For this review, take the finished solid that the model builds, in its own axes (mm). Face numbers are marked on the shaded views. A direction names the side the tool comes from. Coordinates: 2 decimals unless noted, no trailing zeros. Order: outer loops, then holes, each group sorted by start corner. A loop starts at its lowest first (then second) coordinate and runs counter-clockwise, first axis right, second up. Notation, with made-up numbers: (45, -18) -> (53, -18) arc R16 ccw to (53, -3) -> close; hole circle Ø10 at (-24, 32.25). An arc over 180 degrees is marked (long way). Write item = value, one per line. Start each with the question number.
1) Wall thickness on probe 1 along X at (y, z) = (-66, -23.48); probe 2 along Y at (x, z) = (-6, -32); probe 3 along Y at (x, z) = (23, 32): over which ranges is each line inside the solid? List them lowest first. Write a range as [from, to].
2) Consider section B-B on z = -23.48. Give the boundary of the cut face in (x, y).
3) Consider section A-A on x = 25. Give the boundary of the cut face in (y, z).
4) Draft analysis for pull direction Y (two halves, no side actions). For the marked faces 1, 2, 3 and 4, state which applies: +Y half, -Y half, draft (parallel to the pull), parting line (faces both ways), or undercut.
5) Consider section D-D on z = -38.5. Give the boundary of the cut face in (x, y).
6) Machinability: for the marked faces 5, 6 and 7, which of the approach directions +Z, -Z, +X, -X, +Y, -Y give a long, thin tool a straight path to every point of the face, cutting with its end or side? Answer none if there is none.
7) Insertion check: pin 1 Ø3 at (x, z) = (7.5, 7.5) entering from -Y; pin 2 Ø1.6 at (y, z) = (-21, -52.5) entering from +X; pin 3 Ø5.5 at (x, y) = (0, -77) entering from -Z. Each pin has a flat end and moves straight along its axis. Give the tip position at first contact, or say it passes through.
8) Consider section C-C on y = -77. Give the boundary of the cut face in (x, z).
from build123d import *

# Parameters (mm, degrees)
SKETCH1_W           = 68
SKETCH1_H           = 107
BOSS_EXTRUDE1_DEPTH = 2
SKETCH2_W           = 68
SKETCH2_H           = 2
BOSS_EXTRUDE2_DEPTH = 67
CUT_EXTRUDE2_REACH  = 132.744
SKETCH4_W           = 11.5
SKETCH4_H           = 15
SKETCH4_W_2         = 38
SKETCH4_H_2         = 21
SKETCH5_W           = 68
SKETCH5_H           = 2
BOSS_EXTRUDE3_DEPTH = 51
SKETCH6_W           = 68
SKETCH6_H           = 2
BOSS_EXTRUDE4_DEPTH = 15
BOSS_EXTRUDE5_DEPTH = 1.5
CUT_EXTRUDE4_REACH  = 96.449
SKETCH9_R           = 1.75
FILLET1_R           = 1.5
FILLET2_R           = 3
FILLET3_R           = 1.5
FILLET4_R           = 3
FILLET5_R           = 1.5
FILLET6_R           = 3
CUT_EXTRUDE5_REACH  = 106.585
SKETCH10_R          = 1.75
CHAMFER1_SIZE       = 2


with BuildPart() as part:
    # Sketch1 → Boss-Extrude1 (new body)
    with BuildSketch(Plane(origin=(0, 0, 0), x_dir=(1, 0, 0), z_dir=(0, 1, 0))):
        Rectangle(SKETCH1_W, SKETCH1_H)
    extrude(amount=BOSS_EXTRUDE1_DEPTH)

    # Sketch2 → Boss-Extrude2 (add)
    with BuildSketch(Plane.XZ):
        with Locations((0, -52.5)):
            Rectangle(SKETCH2_W, SKETCH2_H)
    extrude(amount=BOSS_EXTRUDE2_DEPTH)

    # Sketch4 → Cut-Extrude2 (cut, up to next)
    with BuildSketch(Plane(origin=(0, 0, -53.5), x_dir=(-1, 0, 0), z_dir=(0, 0, -1)), mode=Mode.PRIVATE) as cut_extrude2_sk1:
        with Locations((-25.25, -28)):
            Rectangle(SKETCH4_W, SKETCH4_H)
    cut_extrude2_tool1 = extrude(cut_extrude2_sk1.sketch, amount=-CUT_EXTRUDE2_REACH, mode=Mode.PRIVATE) & part.part
    # Sketch4 → Cut-Extrude2 (cut, up to next)
    with BuildSketch(Plane(origin=(0, 0, -53.5), x_dir=(-1, 0, 0), z_dir=(0, 0, -1)), mode=Mode.PRIVATE) as cut_extrude2_sk2:
        with Locations((9.546940835, -25.7)):
            Rectangle(SKETCH4_W_2, SKETCH4_H_2)
    cut_extrude2_tool2 = extrude(cut_extrude2_sk2.sketch, amount=-CUT_EXTRUDE2_REACH, mode=Mode.PRIVATE) & part.part
    add(cut_extrude2_tool1.solids().sort_by_distance((25.25, -28, -53.5))[0], mode=Mode.SUBTRACT)
    add(cut_extrude2_tool2.solids().sort_by_distance((-9.546941, -25.7, -53.5))[0], mode=Mode.SUBTRACT)

    # Sketch5 → Boss-Extrude3 (add)
    with BuildSketch(Plane.XY.offset(-51.5)):
        with Locations((0, -66)):
            Rectangle(SKETCH5_W, SKETCH5_H)
    extrude(amount=BOSS_EXTRUDE3_DEPTH)

    # Sketch6 → Boss-Extrude4 (add)
    with BuildSketch(Plane.XZ.offset(67)):
        with Locations((0, -1.5)):
            Rectangle(SKETCH6_W, SKETCH6_H)
    extrude(amount=BOSS_EXTRUDE4_DEPTH)

    # Sketch8 → Boss-Extrude5 (add)
    with BuildSketch(Plane(origin=(0, 2, 0), x_dir=(1, 0, 0), z_dir=(0, 1, 0))):
        Polygon((-34.8, 50.5), (-34, 50.5), (-34, -53.5), (34, -53.5), (34, 50.5), (34.8, 50.5), (34.8, -54.3), (-34.8, -54.3), align=None)
    extrude(amount=-BOSS_EXTRUDE5_DEPTH)

    # Sketch9 → Cut-Extrude4 (cut, up to next)
    with BuildSketch(Plane.XZ.offset(67), mode=Mode.PRIVATE) as cut_extrude4_sk1:
        with Locations(Location((-25, -23.48, 0), (0, 0, 270))):
            Circle(SKETCH9_R)
    cut_extrude4_tool1 = extrude(cut_extrude4_sk1.sketch, amount=-CUT_EXTRUDE4_REACH, mode=Mode.PRIVATE) & part.part
    # Sketch9 → Cut-Extrude4 (cut, up to next)
    with BuildSketch(Plane.XZ.offset(67), mode=Mode.PRIVATE) as cut_extrude4_sk2:
        with Locations(Location((25, -23.48, 0), (0, 0, 270))):
            Circle(SKETCH9_R)
    cut_extrude4_tool2 = extrude(cut_extrude4_sk2.sketch, amount=-CUT_EXTRUDE4_REACH, mode=Mode.PRIVATE) & part.part
    add(cut_extrude4_tool1.solids().sort_by_distance((-25, -67, -23.48))[0], mode=Mode.SUBTRACT)
    add(cut_extrude4_tool2.solids().sort_by_distance((25, -67, -23.48))[0], mode=Mode.SUBTRACT)

    # Fillet1
    fillet1_edges = [part.edges().sort_by_distance(p)[0] for p in [
        (0, -67, -2.5),
    ]]
    fillet(fillet1_edges, radius=FILLET1_R)

    # Fillet2
    fillet2_edges = [part.edges().sort_by_distance(p)[0] for p in [
        (0, -65, -0.5),
    ]]
    fillet(fillet2_edges, radius=FILLET2_R)

    # Fillet3
    fillet3_edges = [part.edges().sort_by_distance(p)[0] for p in [
        (0, -65, -51.5),
    ]]
    fillet(fillet3_edges, radius=FILLET3_R)

    # Fillet4
    fillet4_edges = [part.edges().sort_by_distance(p)[0] for p in [
        (0, -67, -53.5),
    ]]
    fillet(fillet4_edges, radius=FILLET4_R)

    # Fillet5
    fillet5_edges = [part.edges().sort_by_distance(p)[0] for p in [
        (0, 0, -51.5),
    ]]
    fillet(fillet5_edges, radius=FILLET5_R)

    # Fillet6
    fillet6_edges = [part.edges().sort_by_distance(p)[0] for p in [
        (0, 2, -53.5),
    ]]
    fillet(fillet6_edges, radius=FILLET6_R)

    # Sketch10 → Cut-Extrude5 (cut, up to next)
    with BuildSketch(Plane.XY.offset(-0.5), mode=Mode.PRIVATE) as cut_extrude5_sk1:
        with Locations((0, -77)):
            Circle(SKETCH10_R)
    cut_extrude5_tool1 = extrude(cut_extrude5_sk1.sketch, amount=-CUT_EXTRUDE5_REACH, mode=Mode.PRIVATE) & part.part
    add(cut_extrude5_tool1.solids().sort_by_distance((0, -77, -0.5))[0], mode=Mode.SUBTRACT)

    # Chamfer1
    chamfer1_edges = [part.edges().sort_by_distance(p)[0] for p in [
        (-34, -82, -1.5),
        (34, -82, -1.5),
    ]]
    chamfer(chamfer1_edges, length=CHAMFER1_SIZE)


solid = part.part
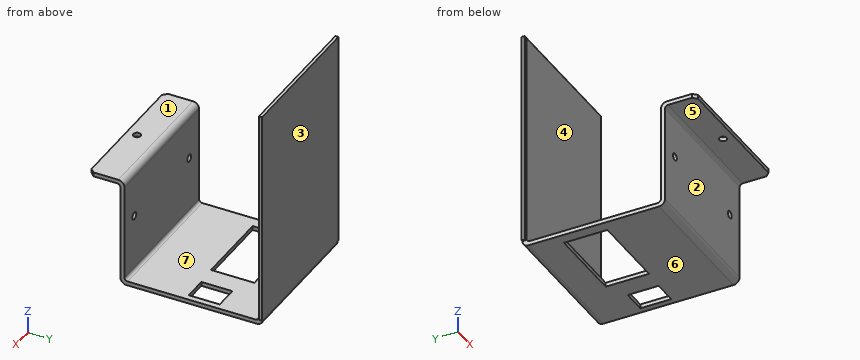
Answer sheet:
q1.probe_1 = [-34, -26.75], [-23.25, 23.25], [26.75, 34]
q1.probe_2 = [-67, -65], [0, 2]
q1.probe_3 = [0, 2]
q2.outline = (-34.8, 0.5) -> (-34, 0.5) -> (-34, 0) -> (34, 0) -> (34, 0.5) -> (34.8, 0.5) -> (34.8, 2) -> (-34.8, 2) -> close; (-34, -67) -> (-26.75, -67) -> (-26.75, -65) -> (-34, -65) -> close; (-23.25, -67) -> (23.25, -67) -> (23.25, -65) -> (-23.25, -65) -> close; (26.75, -67) -> (34, -67) -> (34, -65) -> (26.75, -65) -> close
q3.outline = (-82, -2.5) -> (-68.5, -2.5) arc R1.5 cw to (-67, -4) -> (-67, -21.73) -> (-65, -21.73) -> (-65, -3.5) arc R3 ccw to (-68, -0.5) -> (-82, -0.5) -> close; (-67, -50.5) arc R3 ccw to (-64, -53.5) -> (-35.5, -53.5) -> (-35.5, -51.5) -> (-63.5, -51.5) arc R1.5 cw to (-65, -50) -> (-65, -25.23) -> (-67, -25.23) -> close; (-20.5, -53.5) -> (-1, -53.5) arc R3 ccw to (2, -50.5) -> (2, 54.3) -> (0.5, 54.3) -> (0.5, 53.5) -> (0, 53.5) -> (0, -50) arc R1.5 cw to (-1.5, -51.5) -> (-20.5, -51.5) -> close
q4.face_1 = draft
q4.face_2 = -Y half
q4.face_3 = +Y half
q4.face_4 = undercut
q5.outline = (-34.8, 0.5) -> (-34, 0.5) -> (-34, 0) -> (34, 0) -> (34, 0.5) -> (34.8, 0.5) -> (34.8, 2) -> (-34.8, 2) -> close; (-34, -67) -> (34, -67) -> (34, -65) -> (-34, -65) -> close
q6.face_5 = -Z, +X, -X, -Y
q6.face_6 = -Z, +X, -X, +Y, -Y
q6.face_7 = +Z, +X, -X
q7.pin_1 = 0
q7.pin_2 = 34
q7.pin_3 = -2.5
q8.outline = (-34, -2.5) -> (-1.75, -2.5) -> (-1.75, -0.5) -> (-34, -0.5) -> close; (1.75, -2.5) -> (34, -2.5) -> (34, -0.5) -> (1.75, -0.5) -> close
